from build123d import *

# Parameters (mm, degrees)
F0_W     = 308.2244545221
F0_H     = 149.8168706894
F1_DEPTH = 127
F3_T     = -2.54
F2_W     = 308.2244545221
F2_H     = 149.8168706894
F4_DEPTH = 12.7
F5_DEPTH = 12.7
F6_DEPTH = 12.7
F7_DEPTH = 12.7
F8_R     = 5.08
F9_R     = 5.08
F10_R    = 5.08
F11_R    = 5.08
F12_R    = 5.08


with BuildPart() as f1:
    # F0 (on Top) → F1 (new body)
    with BuildSketch(Plane.XY):
        with Locations((1.3804957271, -1.0464191437)):
            Rectangle(F0_W, F0_H)
    extrude(amount=F1_DEPTH)

    # F3
    f3_openings = [f1.faces().sort_by_distance(p)[0] for p in [
        (1.380496, -75.954854, 63.5),
    ]]
    offset(amount=F3_T, openings=f3_openings)

    # F2 (on face) → F4 (join)
    with BuildSketch(Plane.XY.offset(127)):
        with Locations((1.3804957271, -1.0464191437)):
            Rectangle(F2_W, F2_H)
    extrude(amount=F4_DEPTH)

    # F5 (add): a face of the model
    f5_faces = [f1.faces().sort_by_distance(p)[0] for p in [
        (155.4927229881, -1.0464191437, 69.85),
    ]]
    extrude(f5_faces, amount=F5_DEPTH)

    # F6 (add): a face of the model
    f6_faces = [f1.faces().sort_by_distance(p)[0] for p in [
        (-152.731731534, -1.0464191437, 69.85),
    ]]
    extrude(f6_faces, amount=F6_DEPTH)

    # F0 (on Top) → F7 (join)
    with BuildSketch(Plane.XY):
        with Locations((1.3804957271, -1.0464191437)):
            Rectangle(F0_W, F0_H)
    extrude(amount=F7_DEPTH)

    # F8
    f8_edges = [f1.edges().sort_by_distance(p)[0] for p in [
        (-165.431732, -1.046419, 139.7),
        (-165.431732, -1.046419, 0),
        (168.192723, -1.046419, 139.7),
        (168.192723, -1.046419, 0),
    ]]
    fillet(f8_edges, radius=F8_R)

    # F9
    f9_edges = [f1.edges().sort_by_distance(p)[0] for p in [
        (1.380496, 73.862016, 139.7),
    ]]
    fillet(f9_edges, radius=F9_R)

    # F10
    f10_edges = [f1.edges().sort_by_distance(p)[0] for p in [
        (-150.191732, -75.954854, 68.58),
        (1.380496, -75.954854, 12.7),
        (1.380496, -75.954854, 124.46),
        (152.952723, -75.954854, 68.58),
    ]]
    fillet(f10_edges, radius=F10_R)

    # F11
    f11_edges = [f1.edges().sort_by_distance(p)[0] for p in [
        (1.380496, -75.954854, 139.7),
    ]]
    fillet(f11_edges, radius=F11_R)

    # F12
    f12_edges = [f1.edges().sort_by_distance(p)[0] for p in [
        (1.380496, 71.322016, 12.7),
        (-150.191732, 71.322016, 68.58),
        (1.380496, 71.322016, 124.46),
        (152.952723, 71.322016, 68.58),
    ]]
    fillet(f12_edges, radius=F12_R)


solid = f1.part
Could you check a few things on this model? Use its own coordinates, in mm. A direction names the side the tool comes from. Give positions to 0.01 mm unless a question says otherwise; leave off trailing zeros. Loops run counter-clockwise (first coordinate to the right, second up) from the corner with the lowest first, then second, coordinate; pieces in that order, holes last. Notation, with made-up numbers: M 50,-8 L 74,-8 A8 ccw 74,4 Z; hole C 79.25,27.25 d2. An arc over 180 degrees is marked long. Answer as a JSON object with one key per item and string values.
Q1. Suppose I cut it at C-C, the plane x = 23. List the corners of the cut face in (y, z) for me.
Values found:
{"outline": "M -75.95,5.08 A5.08 ccw -70.87,0 L 68.78,0 A5.08 ccw 73.86,5.08 L 73.86,134.62 A5.08 ccw 68.78,139.7 L -70.87,139.7 A5.08 ccw -75.95,134.62 L -75.95,129.54 A5.08 ccw -70.87,124.46 L 66.24,124.46 A5.08 cw 71.32,119.38 L 71.32,17.78 A5.08 cw 66.24,12.7 L -70.87,12.7 A5.08 ccw -75.95,7.62 Z"}
Q2. For faces 4 (the flat face through (-1, 71.322, 68)), 5 (the flat face through (-1, 73.862, 69)), which set-ups out of +Z, -Z, +X, -X, +Y, -Y let a thin tool reach every point of the face, with its end or its side?
Values found:
{"face 4": "-Y", "face 5": "+Z, -Z, +X, -X, +Y"}
Q3. If I drill on probe 1 along X at (y, z) = (-15.5, 41); probe 2 along Z at (x, y) = (-138, -4); probe 3 along Y at (x, z) = (-74.5, 92), over which ranges is the centre line in solid material (lowest first)? Write a range as [from, to].
Values found:
{"probe 1": "x = [-165.43, -150.19], [152.95, 168.19]", "probe 2": "z = [0, 12.7], [124.46, 139.7]", "probe 3": "y = [71.32, 73.86]"}
Q4. Suppose I cut it at B-B, the plane z = 40.5. List the corners of the cut face in (x, y) for me.
Values found:
{"outline": "M -165.43,-70.87 A5.08 ccw -160.35,-75.95 L -155.27,-75.95 A5.08 ccw -150.19,-70.87 L -150.19,66.24 A5.08 cw -145.11,71.32 L 147.87,71.32 A5.08 cw 152.95,66.24 L 152.95,-70.87 A5.08 ccw 158.03,-75.95 L 163.11,-75.95 A5.08 ccw 168.19,-70.87 L 168.19,68.78 A5.08 ccw 163.11,73.86 L -160.35,73.86 A5.08 ccw -165.43,68.78 Z"}
Q5. Suppose I cut it at A-A, the plane y = -37. List the corners of the cut face in (x, z) for me.
Values found:
{"outline": "M -165.43,5.08 A5.08 ccw -160.35,0 L 163.11,0 A5.08 ccw 168.19,5.08 L 168.19,134.62 A5.08 ccw 163.11,139.7 L -160.35,139.7 A5.08 ccw -165.43,134.62 Z; hole M -150.19,12.7 L 152.95,12.7 L 152.95,124.46 L -150.19,124.46 Z"}
Q6. If we mould it in two halves opening along X, with no side actions, what happens to faces 1 (the flat face through (-150.192, -3, 68)), 2 (the flat face through (-1, 0, 0)), 3 (the flat face through (168.193, -2, 69))? For each: pulls with the +X half, pulls with the -X half, needs draft (parallel to the pull), parting line crosses it, or undercut.
Values found:
{"face 1": "undercut", "face 2": "needs draft", "face 3": "pulls with the +X half"}
